Autodesk Inventor part; units mm, degrees
ref_plane "YZ Plane" through (0, 0, 0) normal (1, 0, 0) x (0, 1, 0)
ref_plane "XZ Plane" through (0, 0, 0) normal (0, 1, 0) x (-1, 0, 0)
ref_plane "XY Plane" through (0, 0, 0) normal (0, 0, 1) x (1, 0, 0)
sketch "Szkic1" plane through (0, 0, 0) normal (0, 0, 1) x (1, 0, 0)
  line L0 (-41.2071, 0) -> (178.5929, 0)
  line L1 (0, -47.06) -> (0, 194.51)
  line L2 (0, 0) -> (0, 6) construction
  line L3 (0, 6) -> (-4.1, 6)
  line L4 (-4.1, 6) -> (-4.8071, 5.2929)
  line L5 (-4.1, 6) -> (-3.1, 6) construction
  line L6 (0, 0) -> (-4.8071, 0) construction
  line L7 (-4.8071, 0) -> (-4.8071, 3) construction
  line L8 (-4.8071, 3) -> (-4.8071, 5.2929)
  line L9 (-4.8071, 3) -> (-9.8071, 3)
  line L10 (-9.8071, 3) -> (-9.8071, 160)
  line L11 (-9.8071, 3) -> (147.1929, 3) construction
  line L12 (-9.8071, 160) -> (0, 160)
  line L13 (0, 160) -> (0, 6)
  dimension "d0" = 6
  dimension "d1" = 4.1
  dimension "d5" = 1
  dimension "d6" = 135
  dimension "d7" = 3
  dimension "d8" = 5
  dimension "d9" = 157
  dimension "d10" = 90
revolve "Obrót1" add sketch "Szkic1" angle 360 about axis through (-10, 0, 0) along (1, 0, 0)
sketch "Szkic2" plane through (-9.8071, 0, 0) normal (-1, 0, 0) x (0, 0, 1)
  line L0 (0, 0) -> (11, 0) construction
  circle A0 centre (11, 0) radius 1.55
  circle A1 centre (7.7782, 7.7782) radius 1.55
  circle A2 centre (0, 11) radius 1.55
  circle A3 centre (-7.7782, 7.7782) radius 1.55
  circle A4 centre (-11, 0) radius 1.55
  circle A5 centre (-7.7782, -7.7782) radius 1.55
  circle A6 centre (0, -11) radius 1.55
  circle A7 centre (7.7782, -7.7782) radius 1.55
  circle A8 centre (0, 0) radius 14
  circle A9 centre (0, 0) radius 5.05
  line L1 (5.8312, 0) -> (2.9156, -5.05)
  line L2 (2.9156, 5.05) -> (5.8312, 0)
  line L3 (-2.9156, 5.05) -> (2.9156, 5.05)
  line L4 (-5.8312, 0) -> (-2.9156, 5.05)
  line L5 (-2.9156, -5.05) -> (-5.8312, 0)
  line L6 (2.9156, -5.05) -> (-2.9156, -5.05)
  point P0 (0, -5.05)
  dimension "d21" = 10.1
  dimension "d12" = 11
  dimension "d13" = 3.1
  dimension "d16" = 360
  dimension "d20" = 28
  dimension "d26" = 360
extrude "Wyciągnięcie proste1" cut sketch "Szkic2" against normal through all contours A0 | A1 | A2 | A3 | A4 | A5 | A6 | A7
extrude "Wyciągnięcie proste2" add sketch "Szkic2" along normal blind 10
fillet "Zaokrąglenie1" radius 10 1 edges at (-9.8071, 0, -14)
Work out the finished part from the listing and answer in its coordinate system (mm). A direction names the side the tool comes from. Give positions to 0.01 mm unless a question says otherwise; leave off trailing zeros. Order: outer loops, then holes, each group sorted by start corner. A loop starts at its lowest first (then second) coordinate and runs counter-clockwise, first axis right, second up. Notation, with made-up numbers: (-37, 60.5) - (6, 60.5) arc R21 ccw to (6, 94.5) - close; hole circle Ø5 at (21, 20.25). An arc over 180 degrees is marked (long way). Answer as CSV lines item,"result". Start each with the question number.
Q1. The part is cut by section B-B (z = 71). Write down the section's boundary in (x, y), then the cut area to 3 significant figures.
Q2. Find the intervals of material crossed by L1, parallel to Y at x = -11.25, z = -7.5; L2, parallel to X at y = -78, z = 45.5; L3, parallel to Y at x = -13, z = -11, in increasing order. Write a range as [from, to].
Q3. The mould has two halves that part along Z. Classify faces 4 (the face through (-4.835, -34.685, -156.195)), 5 (the face through (-2, -6, 0)), 6 (the face through (-19.807, -6, 0)): +Z half, -Z half, draft (parallel to the pull), parting line (faces both ways), or undercut.
Q4. For faces 1 (the face through (-4.807, 2.3, -2.3)), 2 (the face through (0, 33, 2)), 3 (the face through (-9.807, 2, -3)), determine the directions among +Z, -Z, +X, -X, +Y, -Y from which every point of the face is accessible in a straight line to the end or side of a thin tool.
Q5. The part is cut by section C-C (y = 41). Write down the section's boundary in (x, z), then the cut area to 3 significant figures.
Q6. Given pin 1 Ø4 at (x, y) = (-16, 14) entering from -Z; pin 2 Ø2 at (x, z) = (-4.5, -64) entering from -Y; pin 3 Ø4 at (y, z) = (0, -11) entering from -X; pin 4 Ø7 at (y, z) = (0, 0) entering from -X, each flat-ended and moving along its own axis, determine where each tip first touches the part or whether it passes through.
Q7. The part is cut by section A-A (x = -14.75). Give the number of separate pieces and of enclosed holes in the cut face, then the cut area to 3 significant figures.
Check result:
1,outline,"(-9.81, -143.38) - (0, -143.38) - (0, 143.38) - (-9.81, 143.38) - close"
1,area,"2,810 mm²"
2,L1,"y = [-17.27, -9.3], [-6.25, 6.25], [9.3, 17.27]"
2,L2,"x = [-9.81, 0]"
2,L3,"y = [-12.53, -1.55], [1.55, 12.53]"
3,face 4,"parting line"
3,face 5,"undercut"
3,face 6,"draft"
4,face 1,"+X"
4,face 2,"+Z, -Z, +X, +Y, -Y"
4,face 3,"-X"
5,outline,"(-9.81, -154.66) - (0, -154.66) - (0, 154.66) - (-9.81, 154.66) - close"
5,area,"3,030 mm²"
6,pin 1,"stops at z = -9.04"
6,pin 2,"stops at y = -147.07"
6,pin 3,"stops at x = -19.81"
6,pin 4,"stops at x = -9.81"
7,separate pieces,"1"
7,enclosed holes,"9"
7,area,"594 mm²"
